Read the model definition and answer for the solid it produces. Units are mm, in the model's axes. Face numbers are marked on the shaded views. A direction names the side the tool comes from. Round coordinates to 2 decimals unless told otherwise and drop trailing zeros. Loops run counter-clockwise (first coordinate to the right, second up) from the corner with the lowest first, then second, coordinate; pieces in that order, holes last. Notation, with made-up numbers: M 52.25,-27 L 96.25,-27 A6 ccw 96.25,-17 Z; hole C -34,17 d7. An arc over 180 degrees is marked long. Answer as CSV lines item,"result".
Autodesk Inventor part; units mm, degrees
ref_plane "Work Plane1" through (12.5, 0, 0) normal (1, 0, 0) x (0, 1, 0)
ref_plane "XZ Plane" through (0, 0, 0) normal (0, 1, 0) x (-1, 0, 0)
ref_plane "XY Plane" through (0, 0, 0) normal (0, 0, 1) x (1, 0, 0)
sketch "Sketch1" plane through (0, 0, 0) normal (0, 1, 0) x (-1, 0, 0)
  circle A0 centre (0, 0) radius 7.5
  circle A1 centre (0, 0) radius 3
  dimension "d0" = 15
  dimension "d1" = 6
extrude "Extrusion1" add sketch "Sketch1" along normal blind 18
sketch "Sketch2" plane through (0, 18, 0) normal (0, 1, 0) x (1, 0, 0)
  circle A0 centre (0, 0) radius 3
  circle A1 centre (0, 0) radius 2.75
  circle A2 centre (0, 0) radius 4
  dimension "d4" = 5.5
  dimension "d5" = 8
extrude "Extrusion2" add sketch "Sketch2" along normal blind 7 contours A2
fillet "Fillet1" radius 6 1 edges at (-4, 18, 0)
fillet "Fillet2" radius 6 2 edges at (0, 18, -7.5) (0, 18, 7.5)
ref_plane "Work Plane1" through (12.5, 0, 0) normal (1, 0, 0) x (0, 1, 0)
mirror "Mirror1" about plane through (12.5, 0, 0) normal (1, 0, 0) of "Extrusion1", "Extrusion2", "Fillet1", "Fillet2"
sketch "Sketch3" plane through (0, 0, 0) normal (0, 1, 0) x (-1, 0, 0)
  circle A0 centre (-25, 0) radius 3
  line L0 (-25, 0) -> (-25, 3)
  line L1 (-25, 0) -> (-25, -3)
  line L2 (0, 0) -> (0, -3)
  circle A1 centre (0, 0) radius 3
  line L3 (0, 0) -> (0, 3)
  line L4 (-25, 3) -> (0, 3)
  line L5 (0, 3) -> (0, 7.5)
  line L6 (0, 7.5) -> (-25, 7.5)
  line L7 (-25, 7.5) -> (-25, 3)
  line L8 (-25, -3) -> (0, -3)
  line L9 (0, -3) -> (0, -7.5)
  line L10 (0, -7.5) -> (-25, -7.5)
  line L11 (-25, -7.5) -> (-25, -3)
  point P0 (0, -3)
  point P1 (0, 3)
  dimension "d11" = 25
  dimension "d12" = 4.5
  dimension "d13" = 25
  dimension "d14" = 4.5
extrude "Extrusion3" add sketch "Sketch3" along normal blind 13 contours A0 L4 A1 L8 | L7 L6 L5 L4 | L8 L9 L10 L11
sketch "Sketch4" plane through (0, 0, 7.5) normal (0, 0, 1) x (1, 0, 0)
  line L0 (25, 13) -> (0, 13)
  circle A0 centre (12.5, 5) radius 3
  line L1 (0, 0) -> (25, 0)
  line L2 (0, 0) -> (0, 13)
  point P0 (25, 15)
  point P1 (0, 15)
  dimension "d18" = 6
  dimension "d21" = 5
  dimension "d22" = 12.5
extrude "Extrusion4" cut sketch "Sketch4" against normal through all
properties part number "4mm_Roller_Spacer_extended"
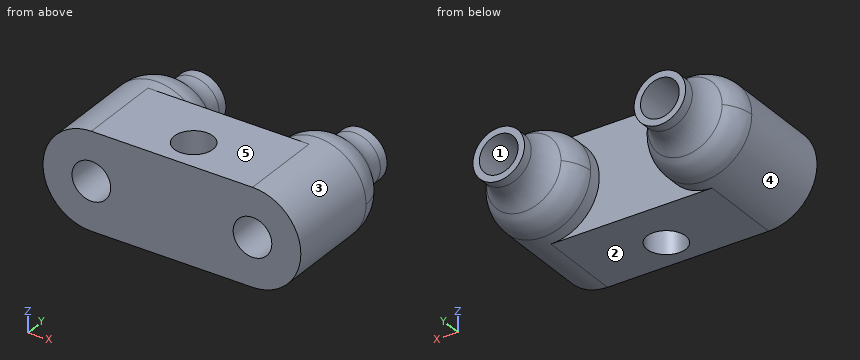
1) Determine the mould class of the marked faces 1, 2 and 3 for opening direction Z: released by +Z, released by -Z, zero draft, split by the parting line, or undercut.
Evaluation:
face 1,"undercut"
face 2,"released by -Z"
face 3,"split by the parting line"
2) Straight lines are drawn through the part: line 1 (Y direction, x = 12.5, z = 4); line 2 (Z direction, x = 0, y = 6.25); line 3 (X direction, y = 3, z = -0.25). For each, find the intervals that lie inside material, in ascending order.
Evaluation:
line 1,"y = 0 to 2, 8 to 13"
line 2,"z = -7.5 to -3, 3 to 7.5"
line 3,"x = -7.5 to -2.99, 2.99 to 10.26, 14.74 to 22.01, 27.99 to 32.5"
3) A tool of negligible diameter and unlimited length cuts with its end or side. For the marked faces 4 and 5, from which of +Z, -Z, +X, -X, +Y, -Y can it reach the whole face along a straight path? Write none if from no direction.
Evaluation:
face 4,"+Y"
face 5,"+Z, +X, -X, +Y, -Y"
4) Find section A-A, the plane y = 5. Give the vertices of the cut face in (x, z).
Evaluation:
outline,"M 0,-7.5 L 9.5,-7.5 L 9.5,7.5 L 0,7.5 A7.5 ccw Z; M 15.5,-7.5 L 25,-7.5 A7.5 ccw 25,7.5 L 15.5,7.5 Z; hole C 0,0 d6; hole C 25,0 d6"
5) Find section D-D, the plane y = 20.5. Give the vertices of the cut face in (x, z).
Evaluation:
outline,"C 0,0 d9.56; C 25,0 d9.56; hole C 0,0 d6; hole C 25,0 d6"
6) Each of these flat-tipped pins is pushed along its axis until it touches: P1, Ø4, axis at y = 10, z = -4, coming from the +X side; P2, Ø1.5, axis at y = 19.5, z = -3, coming from the -X side; P3, Ø3, axis at y = 11, z = -4, coming from the -X side. Where does it stop, or does it pass through?
Evaluation:
P1,"stops at x = 32.23"
P2,"stops at x = -5.49"
P3,"stops at x = -7.07"
7) Find section C-C, the plane y = 10. Give the vertices of the cut face in (x, z).
Evaluation:
outline,"M 0,-7.5 L 25,-7.5 A7.5 ccw 25,7.5 L 0,7.5 A7.5 ccw Z; hole C 0,0 d6; hole C 25,0 d6"
8) Find section B-B, the plane x = 12.5. Give the vertices of the cut face in (y, z).
Evaluation:
outline,"M 0,-7.5 L 2,-7.5 L 2,7.5 L 0,7.5 Z; M 8,-7.5 L 13,-7.5 L 13,7.5 L 8,7.5 Z"
